```python
from build123d import *

# Parameters (mm, degrees)
BOSS_EXTRUDE1_DEPTH        = 508
F_1_2_0_5_DIAMETER_HOLE1_D = 12.7
CUT_EXTRUDE3_REACH         = 52.8


with BuildPart() as part:
    # Sketch1 → Boss-Extrude1 (new body, symmetric)
    with BuildSketch(Plane.XY):
        with BuildLine():
            Line((12.7, 0), (38.1, 0))
            ThreePointArc((38.1, 0), (47.080256121, 3.719743879), (50.8, 12.7))
            Line((50.8, 12.7), (50.8, 38.1))
            ThreePointArc((50.8, 38.1), (47.080256121, 47.080256121), (38.1, 50.8))
            Line((38.1, 50.8), (12.7, 50.8))
            ThreePointArc((12.7, 50.8), (3.719743879, 47.080256121), (0, 38.1))
            Line((0, 38.1), (0, 12.7))
            ThreePointArc((0, 12.7), (3.719743879, 3.719743879), (12.7, 0))
        make_face()
        with BuildLine():
            Line((12.7, 6.35), (38.1, 6.35))
            ThreePointArc((38.1, 6.35), (42.590128061, 8.209871939), (44.45, 12.7))
            Line((44.45, 12.7), (44.45, 38.1))
            ThreePointArc((44.45, 38.1), (42.590128061, 42.590128061), (38.1, 44.45))
            Line((38.1, 44.45), (12.7, 44.45))
            ThreePointArc((12.7, 44.45), (8.209871939, 42.590128061), (6.35, 38.1))
            Line((6.35, 38.1), (6.35, 12.7))
            ThreePointArc((6.35, 12.7), (8.209871939, 8.209871939), (12.7, 6.35))
        make_face(mode=Mode.SUBTRACT)
    extrude(amount=BOSS_EXTRUDE1_DEPTH, both=True)

    # 1/2 (0.5) Diameter Hole1 (through all)
    with Locations(Plane(origin=(0, 50.8, 0), x_dir=(-1, 0, 0), z_dir=(0, 1, 0))):
        with Locations((-25.4, -76.2)):
            Hole(F_1_2_0_5_DIAMETER_HOLE1_D / 2)

    # Sketch9 → Cut-Extrude3 (cut, up to next)
    with BuildSketch(Plane.XZ, mode=Mode.PRIVATE) as cut_extrude3_sk1:
        with BuildLine():
            Line((19.05, -488.95), (19.05, -469.9))
            ThreePointArc((19.05, -469.9), (25.4, -463.55), (31.75, -469.9))
            Line((31.75, -469.9), (31.75, -488.95))
            ThreePointArc((31.75, -488.95), (25.4, -495.3), (19.05, -488.95))
        make_face()
    cut_extrude3_tool1 = extrude(cut_extrude3_sk1.sketch, amount=-CUT_EXTRUDE3_REACH, mode=Mode.PRIVATE) & part.part
    add(cut_extrude3_tool1.solids().sort_by_distance((25.4, 0, -479.425))[0], mode=Mode.SUBTRACT)


solid = part.part
```
Verification items for the finished model (mm, model axes). A direction names the side the tool comes from. Round coordinates to 2 decimals unless told otherwise and drop trailing zeros. Loops run counter-clockwise (first coordinate to the right, second up) from the corner with the lowest first, then second, coordinate; pieces in that order, holes last. Notation, with made-up numbers: (-24.75, 21.5) -> (-9.75, 21.5) arc R21 ccw to (-9.75, 40.5) -> close; hole circle Ø10 at (32, 48.25). An arc over 180 degrees is marked (long way). Answer as a JSON object with one key per item and string values.
Q1. Section check B-B (y = 29). Record the boundary of the cut face in (x, z).
Data:
{"outline": "(0, -508) -> (6.35, -508) -> (6.35, 508) -> (0, 508) -> close; (44.45, -508) -> (50.8, -508) -> (50.8, 508) -> (44.45, 508) -> close"}
Q2. Access from +Z, -Z, +X, -X, +Y, -Y to the whole of each face (thin tool, end or side, straight path). Record for faces 4 (the flat face through (25, 0, 7)), 5 (the flat face through (26, 44.45, 7)).
Data:
{"face 4": "+Z, -Z, +X, -X, -Y", "face 5": "+Z, -Z"}
Q3. Draft check along X on faces 1 (the flat face through (50.8, 25, 7)), 2 (the flat face through (46, 27, 508)), 3 (the flat face through (6.35, 26, 7)). Enter one of: pulls with the +X half, pulls with the -X half, needs draft (parallel to the pull), parting line crosses it, or undercut.
Data:
{"face 1": "pulls with the +X half", "face 2": "needs draft", "face 3": "undercut"}
Q4. Scan lines: line 1 (Z direction, x = 25.4, y = 4.5); line 2 (X direction, y = 37, z = 436); line 3 (Z direction, x = 24.5, y = 45). Record each from-to range of solid material in increasing order. Write a range as from..to.
Data:
{"line 1": "z = -508..-495.3, -463.55..-82.55, -69.85..508", "line 2": "x = 0..6.35, 44.45..50.8", "line 3": "z = -508..-82.49, -69.91..508"}
Q5. Section check A-A (z = 446.5). Record the boundary of the cut face in (x, y), then the cut area to 3 significant figures.
Data:
{"outline": "(0, 12.7) arc R12.7 ccw to (12.7, 0) -> (38.1, 0) arc R12.7 ccw to (50.8, 12.7) -> (50.8, 38.1) arc R12.7 ccw to (38.1, 50.8) -> (12.7, 50.8) arc R12.7 ccw to (0, 38.1) -> close; hole (6.35, 12.7) arc R6.35 ccw to (12.7, 6.35) -> (38.1, 6.35) arc R6.35 ccw to (44.45, 12.7) -> (44.45, 38.1) arc R6.35 ccw to (38.1, 44.45) -> (12.7, 44.45) arc R6.35 ccw to (6.35, 38.1) -> close", "area": "1,030 mm2"}
Q6. Go/stop test with flat-tipped pins: P1, Ø1.5, axis at x = 8.5, z = 247, coming from the +Y side; P2, Ø1.9, axis at y = 3, z = -480.5, coming from the +X side; P3, Ø6, axis at x = 43.5, z = 262.5, coming from the +Y side; P4, Ø12, axis at x = 15, y = 25.5, coming from the +Z side. Record where each tip stops, or that it passes through.
Data:
{"P1": "stops at y = 50.32", "P2": "stops at x = 47.3", "P3": "stops at y = 50.57", "P4": "passes through"}
